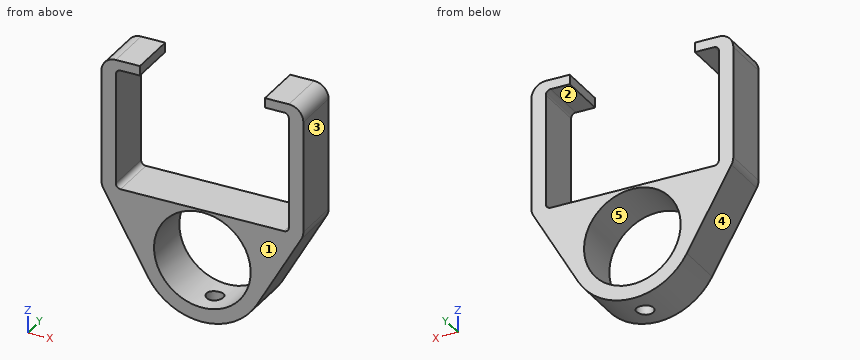
```python
from build123d import *

# Parameters (mm, degrees)
SKETCH_1_R          = 10.05
EXTRUDE_1_DEPTH     = 10
FILLET_1_R          = 3
FILLET_2_R          = 1
SKETCH_2_R          = 1.75
CUT_EXTRUDE_1_DEPTH = 45.127655727


with BuildPart() as part:
    # 草图1 → 凸台-拉伸1 (new body)
    with BuildSketch(Plane(origin=(0, 0, 0), x_dir=(1, 0, 0), z_dir=(0, 1, 0))):
        with BuildLine():
            Line((-11.33930071, 6.459315707), (-21, -10.5))
            Line((-21, -10.5), (-21, -37.5))
            Line((-21, -37.5), (-13, -37.5))
            Line((-13, -37.5), (-13, -35.5))
            Line((-13, -35.5), (-18, -35.5))
            Line((-18, -35.5), (-18, -10.5))
            Line((-18, -10.5), (18, -10.5))
            Line((18, -10.5), (18, -35.5))
            Line((18, -35.5), (13, -35.5))
            Line((13, -35.5), (13, -37.5))
            Line((13, -37.5), (21, -37.5))
            Line((21, -37.5), (21, -10.5))
            Line((21, -10.5), (11.33930071, 6.459315707))
            ThreePointArc((11.33930071, 6.459315707), (0, 13.05), (-11.33930071, 6.459315707))
        make_face()
        with Locations(Location((0, 0, 0), (0, 0, 270))):
            Circle(SKETCH_1_R, mode=Mode.SUBTRACT)
    extrude(amount=EXTRUDE_1_DEPTH)

    # 圆角1
    fillet_1_edges = [part.edges().sort_by_distance(p)[0] for p in [
        (21, 5, 37.5),
        (-21, 5, 37.5),
        (-21, 5, 10.5),
        (21, 5, 10.5),
    ]]
    fillet(fillet_1_edges, radius=FILLET_1_R)

    # 圆角2
    fillet_2_edges = [part.edges().sort_by_distance(p)[0] for p in [
        (18, 5, 10.5),
        (-18, 5, 10.5),
        (-18, 5, 35.5),
        (18, 5, 35.5),
    ]]
    fillet(fillet_2_edges, radius=FILLET_2_R)

    # 草图2 → 切除-拉伸1 (cut, through all)
    with BuildSketch(Plane.XY):
        with Locations(Location((0, 5, 0), (0, 0, 90))):
            Circle(SKETCH_2_R)
    extrude(amount=-CUT_EXTRUDE_1_DEPTH, mode=Mode.SUBTRACT)


solid = part.part
```
The listing builds one solid part. Answer for the finished solid, in the listing's coordinates (mm). Face numbers are marked on the shaded views. A direction names the side the tool comes from. Coordinates: 2 decimals unless noted, no trailing zeros. Write each loop counter-clockwise with the first axis right and the second up, starting at its lowest first coordinate (ties: lowest second). Pieces come first, ordered by that corner, then holes.
Q1. The mould has two halves that part along Z. Classify the marked faces 3, 4 and 5: released by +Z, released by -Z, zero draft, split by the parting line, or undercut.
Returned:
face 3: zero draft
face 4: released by -Z
face 5: undercut
Q2. Section B-B, the plane x = 0 is taken. Write down the section's boundary in (y, z), then the cut area to 3 significant figures.
Returned:
outline: (0, -13.05) - (3.25, -13.05) - (3.25, -10.05) - (0, -10.05) - close; (0, 10.05) - (10, 10.05) - (10, 10.5) - (0, 10.5) - close; (6.75, -13.05) - (10, -13.05) - (10, -10.05) - (6.75, -10.05) - close
area: 24.0 mm2
Q3. Section D-D, the plane x = 7 is taken. Write down the section's boundary in (y, z), then the cut area to 3 significant figures.
Returned:
outline: (0, -11.01) - (10, -11.01) - (10, -7.21) - (0, -7.21) - close; (0, 7.21) - (10, 7.21) - (10, 10.5) - (0, 10.5) - close
area: 70.9 mm2
Q4. Find the intervals of material crossed by line 1 along X through (y, z) = (4.75, 20.5); line 2 along X through (y, z) = (7.75, 6.5); line 3 along Z through (x, y) = (14.5, 2.5), in increasing order.
Returned:
line 1: x = -21 to -18, 18 to 21
line 2: x = -18.72 to -7.67, 7.67 to 18.72
line 3: z = -0.91 to 10.5, 35.5 to 37.5
Q5. Section C-C, the plane z = 0 is taken. Write down the section's boundary in (x, y).
Returned:
outline: (-15.02, 0) - (-10.05, 0) - (-10.05, 10) - (-15.02, 10) - close; (10.05, 0) - (15.02, 0) - (15.02, 10) - (10.05, 10) - close
Q6. Given P1, Ø1, axis at y = 3, z = 36.5, coming from the +X side; P2, Ø2, axis at x = 0, y = 5, coming from the +Z side; P3, Ø2, axis at y = 6.5, z = 36, coming from the -X side, each flat-ended and moving along its own axis, determine where each tip first touches the part or whether it passes through.
Returned:
P1: stops at x = 20.6
P2: stops at z = 10.5
P3: stops at x = -20.96
Q7. Which of the six approach directions +Z, -Z, +X, -X, +Y, -Y give full straight-line access (tool end or side, diameter ignored) to the marked faces 1 and 2?
Returned:
face 1: +Z, -Z, +X, -X, -Y
face 2: +Y, -Y
Q8. Section A-A, the plane y = 2 is taken. Write down the section's boundary in (x, z), then the cut area to 3 significant figures.
Returned:
outline: (-21, 11.29) arc R3 ccw to (-20.61, 9.81) - (-11.34, -6.46) arc R13.05 ccw to (11.34, -6.46) - (20.61, 9.81) arc R3 ccw to (21, 11.29) - (21, 34.5) arc R3 ccw to (18, 37.5) - (13, 37.5) - (13, 35.5) - (17, 35.5) arc R1 cw to (18, 34.5) - (18, 11.5) arc R1 cw to (17, 10.5) - (-17, 10.5) arc R1 cw to (-18, 11.5) - (-18, 34.5) arc R1 cw to (-17, 35.5) - (-13, 35.5) - (-13, 37.5) - (-18, 37.5) arc R3 ccw to (-21, 34.5) - close; hole circle Ø20.1 at (0, 0)
area: 516 mm2
